```python
from build123d import *

# Parameters (mm, degrees)
SKETCH1_R      = 2.6
EXTRUDE1_DEPTH = 5.8
SKETCH2_W      = 2
SKETCH2_H      = 1
FILLET1_R      = 0.5


with BuildPart() as part:
    # Sketch1 → Extrude1 (new body)
    with BuildSketch(Plane(origin=(0, 0, 0), x_dir=(1, 0, 0), z_dir=(0, 1, 0))):
        Polygon((0, -5.773502692), (5, -2.886751346), (5, 2.886751346), (0, 5.773502692), (-5, 2.886751346), (-5, -2.886751346), align=None)
        with Locations(Location((0, 0, 0), (0, 0, 270))):
            Circle(SKETCH1_R, mode=Mode.SUBTRACT)
    extrude(amount=EXTRUDE1_DEPTH)

    # Sketch2 → Cut-Revolve1 (revolve, cut)
    with BuildSketch(Plane.XY, mode=Mode.PRIVATE) as cut_revolve1_sk:
        Polygon((-5, 5.8), (-5, 4.809401077), (-9, 2.5), (-9, 5.8), align=None)
        with Locations((-1, 5.3)):
            Rectangle(SKETCH2_W, SKETCH2_H)
        Polygon((-5, 0), (-9, 0), (-9, 2.309401077), align=None)
    revolve(cut_revolve1_sk.sketch.rotate(Axis((0, 0, 0), (0, 1, 0)), 180), axis=Axis((0, 0, 0), (0, 1, 0)), mode=Mode.SUBTRACT)

    # Fillet1
    fillet1_edges = [part.edges().sort_by_distance(p)[0] for p in [
        (-5, 5.8, 0),
    ]]
    fillet(fillet1_edges, radius=FILLET1_R)


solid = part.part
```
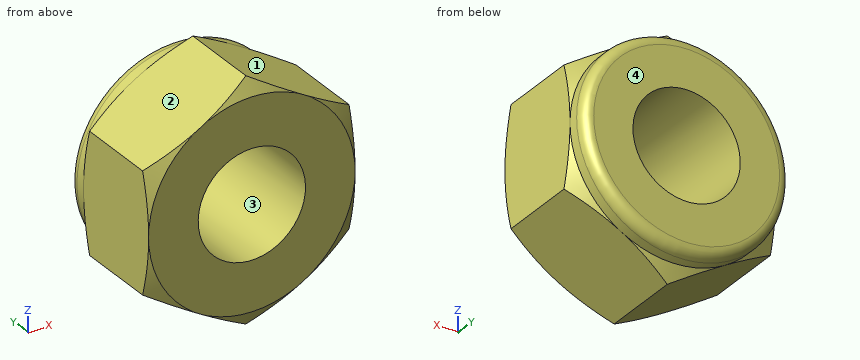
Input: part model. Units: mm. Frame: model coordinates. Face numbers are marked on the shaded views. Give positions to 0.01 mm unless a question says otherwise; leave off trailing zeros. Order: outer loops, then holes, each group sorted by start corner. A loop starts at its lowest first (then second) coordinate and runs counter-clockwise, first axis right, second up. Notation, with made-up numbers: M 66,15.5 L 101,15.5 A13 cw 101,23.5 Z; hole C 39,39.25 d8. An arc over 180 degrees is marked long. One line per question, with ' | ' between items. Start each with the question number.
1. Material intervals for probe 1 along Z at (x, y) = (-0.5, 5.3); probe 2 along Z at (x, y) = (-0.75, 3.5); probe 3 along Z at (x, y) = (4.25, 4.15), sorted ascending. Write a range as [from, to].
2. Pull-direction query (X, two-part tool) for the marked faces 1, 2, 3 and 4; classes: released by +X, released by -X, zero draft, split by the parting line, or undercut.
3. Section query A-A (y = 2.75). Return the cut outline in (x, z), and give its area (3 significant figures).
4. First-contact query: pin 1 Ø1.5 at (x, y) = (-3, 2.5) entering from -Z; pin 2 Ø4.5 at (x, z) = (0, 0) entering from -Y. Flat tips, straight axial feed; report the tip coordinate or a pass-through.
Here are the results:
1) probe 1: [-4.97, -2.55], [2.55, 4.97] | probe 2: [-5.34, -2.49], [2.49, 5.34] | probe 3: [-3.32, 3.32]
2) face 1: released by +X | face 2: released by -X | face 3: undercut | face 4: zero draft
3) outline: M -5,-2.89 L 0,-5.77 L 5,-2.89 L 5,2.89 L 0,5.77 L -5,2.89 Z; hole C 0,0 d5.2 | area: 65.4 mm²
4) pin 1: z = -4.47 | pin 2: through
